Work out the finished part from the listing and answer in its coordinate system (mm). A direction names the side the tool comes from. Coordinates: 2 decimals unless noted, no trailing zeros. Order: outer loops, then holes, each group sorted by start corner. A loop starts at its lowest first (then second) coordinate and runs counter-clockwise, first axis right, second up. Notation, with made-up numbers: M -5.75,60 L 13.25,60 A19 ccw 13.25,64 Z; hole C 25.25,62 d2. An arc over 180 degrees is marked long. Use a Markdown table: item, result.
from build123d import *

# Parameters (mm, degrees)
SKETCH1_R           = 50
BOSS_EXTRUDE1_DEPTH = 5
SKETCH2_R           = 4
BOSS_EXTRUDE2_DEPTH = 20


with BuildPart() as part:
    # Sketch1 → Boss-Extrude1 (new body)
    with BuildSketch(Plane.XY):
        Circle(SKETCH1_R)
    extrude(amount=-BOSS_EXTRUDE1_DEPTH)

    # Sketch2 → Boss-Extrude2 (add)
    with BuildSketch(Plane.XY):
        with Locations((36, 0)):
            Circle(SKETCH2_R)
        with Locations((-18, 31.176914536)):
            Circle(SKETCH2_R)
        with Locations((-18, -31.176914536)):
            Circle(SKETCH2_R)
    extrude(amount=BOSS_EXTRUDE2_DEPTH)


solid = part.part
(1) A cutting plane is placed at B-B (z = -3). Determine the outline of the cut face in (x, y).
Conclusion:
| item | result |
|---|---|
| outline | C 0,0 d100 |
(2) Given P1, Ø6, axis at x = -9.5, z = 2, coming from the -Y side; P2, Ø1, axis at y = -1.5, z = -2, coming from the +X side; P3, Ø8, axis at y = -37, z = 10.5, coming from the -X side; P4, Ø5, axis at x = -10.5, z = 8.5, coming from the -Y side, each flat-ended and moving along its own axis, determine where each tip first touches the part or whether it passes through.
Conclusion:
| item | result |
|---|---|
| P1 | y = -49.47 |
| P2 | x = 49.99 |
| P3 | x = -21.56 |
| P4 | through |
(3) Determine the mould class of faces 1 (the cylindrical face through (32.8, -2.4, 9.9)), 2 (the cylindrical face through (-16.154, -34.726, 9.86)), 3 (the flat face through (36, 0, 20)) for opening direction Y: pulls with the +Y half, pulls with the -Y half, needs draft (parallel to the pull), parting line crosses it, or undercut.
Conclusion:
| item | result |
|---|---|
| face 1 | parting line crosses it |
| face 2 | undercut |
| face 3 | needs draft |
(4) A cutting plane is placed at D-D (z = 13). Determine the outline of the cut face in (x, y), then the cut area to 3 significant figures.
Conclusion:
| item | result |
|---|---|
| outline | C -18,-31.18 d8; C -18,31.18 d8; C 36,0 d8 |
| area | 151 mm2 |
(5) Straight lines are drawn through the part: L1, parallel to Z at x = -25, y = 16.5; L2, parallel to Y at x = -17, z = 17.75; L3, parallel to Y at x = 30.5, z = -3.25. For each, find the intervals that lie inside material, in ascending order.
Conclusion:
| item | result |
|---|---|
| L1 | -5 to 0 |
| L2 | -35.05 to -27.3, 27.3 to 35.05 |
| L3 | -39.62 to 39.62 |
(6) A cutting plane is placed at A-A (y = 0). Determine the outline of the cut face in (x, z), then the cut area to 3 significant figures.
Conclusion:
| item | result |
|---|---|
| outline | M -50,-5 L 50,-5 L 50,0 L 40,0 L 40,20 L 32,20 L 32,0 L -50,0 Z |
| area | 660 mm2 |
(7) Which of the six approach directions +Z, -Z, +X, -X, +Y, -Y give full straight-line access (tool end or side, diameter ignored) to faces 4 (the flat face through (-18, -31, 20)), 5 (the cylindrical face through (-18.867, 27.272, 9.86))?
Conclusion:
| item | result |
|---|---|
| face 4 | +Z, +X, -X, +Y, -Y |
| face 5 | +Z |
(8) A cutting plane is placed at C-C (x = -18). Determine the outline of the cut face in (y, z).
Conclusion:
| item | result |
|---|---|
| outline | M -46.65,-5 L 46.65,-5 L 46.65,0 L 35.18,0 L 35.18,20 L 27.18,20 L 27.18,0 L -27.18,0 L -27.18,20 L -35.18,20 L -35.18,0 L -46.65,0 Z |
